The listing builds one solid part. Answer for the finished solid, in the listing's coordinates (mm). A direction names the side the tool comes from. Coordinates: 2 decimals unless noted, no trailing zeros. Loops run counter-clockwise (first coordinate to the right, second up) from the corner with the lowest first, then second, coordinate; pieces in that order, holes last. Notation, with made-up numbers: M 79.25,10.25 L 114.25,10.25 A24 cw 114.25,44.25 Z; hole C 39,43 d5. An arc over 180 degrees is marked long. Answer as a JSON object with one key per item and string values. Group by question number.
1. For faces 1 (the face through (-0.6, 4, -25)), 2 (the face through (-7.699, 0.285, -25.336)), determine the directions among +Z, -Z, +X, -X, +Y, -Y from which every point of the face is accessible in a straight line to the end or side of a thin tool.
2. A cutting plane is placed at B-B on x = -4. State how many separate pieces and enclosed holes the cut face has, and give its area (3 significant figures).
3. Determine the mould class of faces 3 (the face through (-4, 2, -50)), 4 (the face through (-4, 3, -44)), 5 (the face through (-0.301, 2.521, -0.285)), 6 (the face through (-4, 4, -41)) for opening direction Z: released by +Z, released by -Z, zero draft, split by the parting line, or undercut.
4. A cutting plane is placed at D-D on z = -8. Give the vertices of the cut face in (x, y).
5. Straight lines are drawn through the part: L1, parallel to Z at x = -4, y = 3.35; L2, parallel to X at y = 3.4, z = -4; L3, parallel to Z at x = -4.5, y = 0.95. For each, find the intervals that lie inside material, in ascending order.
6. A cutting plane is placed at A-A on z = -25. Give the vertices of the cut face in (x, y).
7. A cutting plane is placed at C-C on y = 1.9. Give the vertices of the cut face in (x, z), and give its area (3 significant figures).
8. Given pin 1 (0.6 mm diameter, centred on y = 4.5, z = -31.5, fed in from +X); pin 2 (3.5 mm diameter, centred on x = -4, z = -26, fed in from +Y), each flat-ended and moving along its own axis, determine where each tip first touches the part or whether it passes through.
Autodesk Inventor part; units mm, degrees
ref_plane "YZ Plane" through (0, 0, 0) normal (1, 0, 0) x (0, 1, 0)
ref_plane "XZ Plane" through (0, 0, 0) normal (0, 1, 0) x (-1, 0, 0)
ref_plane "XY Plane" through (0, 0, 0) normal (0, 0, 1) x (1, 0, 0)
sketch "스케치1" plane through (0, 0, 0) normal (0, 1, 0) x (-1, 0, 0)
  line L0 (0, 0) -> (8, 0)
  line L1 (8, 0) -> (8, -50)
  line L2 (8, -50) -> (0, -50)
  line L3 (0, -50) -> (0, 0)
  dimension "d0" = 50
  dimension "d1" = 8
extrude "돌출1" add sketch "스케치1" along normal blind 5
sketch "스케치2" plane through (0, 5, 0) normal (0, 1, 0) x (1, 0, 0)
  circle A0 centre (-4, 4) radius 2
  line L0 (-8, 50) -> (-8, 0)
  line L1 (-8, 0) -> (0, 0)
  circle A1 centre (-4, 46) radius 2
  line L2 (0, 0) -> (0, 50)
  line L3 (0, 50) -> (-8, 50)
  dimension "d4" = 4
  dimension "d5" = 4
  dimension "d6" = 4
  dimension "d7" = 4
  dimension "d8" = 4
  dimension "d9" = 4
sketch "스케치3" plane through (0, 0, 0) normal (0, -1, 0) x (1, 0, 0)
  circle A0 centre (-4, -25) radius 1.5
  line L0 (-8, -50) -> (0, -50)
  line L1 (0, -50) -> (0, 0)
  dimension "d10" = 3
  dimension "d11" = 25
  dimension "d12" = 4
extrude "돌출2" cut sketch "스케치2" against normal blind 5 contours A0 | A1
extrude "돌출3" cut sketch "스케치3" against normal blind 5
fillet "모깎기1" radius 1 12 edges at (-8, 5, -25) (-4, 5, 0) (0, 5, -25) (-4, 0, 0) (0, 0, -25) (0, 2.5, 0) (-8, 2.5, 0) (0, 2.5, -50) (-4, 5, -50) (-4, 0, -50) (-8, 2.5, -50) (-8, 0, -25)
fillet "모깎기3" radius 1 4 edges at (-6, 0, -46) (-6, 0, -4) (-6, 5, -4) (-6, 5, -46)
sketch "스케치4" plane through (0, 0, 0) normal (0, -1, 0) x (1, 0, 0)
  point P0 (0, 0)
sketch "스케치5" plane through (0, 5, 0) normal (0, 1, 0) x (1, 0, 0)
  line L0 (-7.5, 9) -> (-0.6, 9)
  line L1 (-0.6, 9) -> (-0.6, 41)
  line L2 (-0.6, 41) -> (-7.5, 41)
  line L3 (-7.5, 41) -> (-7.5, 9)
  line L4 (-4, 1) -> (-7, 1)
  line L5 (-1, 46) -> (-1, 4)
  point P0 (0, 0)
  dimension "d20" = 6.9
  dimension "d21" = 32
  dimension "d22" = 32
  dimension "d23" = 8
  dimension "d24" = 6.5
extrude "돌출4" cut sketch "스케치5" against normal blind 1.3
properties part number "핸들서보"
From the geometry:
{
 "1": {"face 1": "+Y", "face 2": "+Z, -Z, -X, -Y"},
 "2": {"separate pieces": "4", "enclosed holes": "0", "area": "155 mm²"},
 "3": {"face 3": "released by -Z", "face 4": "undercut", "face 5": "released by +Z", "face 6": "undercut"},
 "4": {"outline": "M -8,1 A1 ccw -7,0 L -1,0 A1 ccw 0,1 L 0,4 A1 ccw -1,5 L -7,5 A1 ccw -8,4 Z"},
 "5": {"L1": "z = -50 to -48, -44 to -26.5, -23.5 to -6, -2 to 0", "L2": "x = -8 to -6, -2 to 0", "L3": "z = -50 to -47.94, -44.06 to -26.41, -23.59 to -5.94, -2.06 to 0"},
 "6": {"outline": "M -8,1 A1 ccw -7,0 L -5.5,0 L -5.5,3.7 L -7.5,3.7 L -7.5,4.87 A1 ccw -8,4 Z; M -2.5,0 L -1,0 A1 ccw 0,1 L 0,4 A1 ccw -0.6,4.92 L -0.6,3.7 L -2.5,3.7 Z"},
 "7": {"outline": "M -8,-49 A1 ccw -7,-50 L -1,-50 A1 ccw 0,-49 L 0,-1 A1 ccw -1,0 L -7,0 A1 ccw -8,-1 Z; hole C -4,-46 d4; hole C -4,-4 d4; hole C -4,-25 d3", "area": "367 mm²"},
 "8": {"pin 1": "stops at x = -0.02", "pin 2": "stops at y = 3.7"}
}
